from build123d import *

# Parameters (mm, degrees)
SKETCH2_R           = 5
BOSS_EXTRUDE1_DEPTH = 10


with BuildPart() as part:
    # Sketch2 → Boss-Extrude1 (new body)
    with BuildSketch(Plane(origin=(0, 0, 0), x_dir=(1, 0, 0), z_dir=(0, 1, 0))):
        with BuildLine():
            ThreePointArc((-27.5, -47.631397208), (-14.235047481, -53.125920446), (0, -55))
            add(Edge.make_bspline(
                [(0, -55), (15.821995191, -55.521684642), (37.158196695, -40.15721482), (40.409843735, -11.080588617), (32.003444862, 9.061174356), (19.786389501, 17.600648721), (12.5, 21.650635095)],
                knots=[0, 0, 0, 0, 0.421298926, 0.607822378, 0.766892621, 1, 1, 1, 1], degree=3))
            ThreePointArc((12.5, 21.650635095), (6.470476128, 24.148145657), (0, 25))
            add(Edge.make_bspline(
                [(0, 25), (-8.335191597, 25.135803666), (-23.185209081, 23.848929612), (-40.536245546, 10.608850636), (-52.258549707, -16.198069832), (-41.463092095, -40.172191766), (-27.5, -47.631397208)],
                knots=[0, 0, 0, 0, 0.233107379, 0.392177622, 0.578701074, 1, 1, 1, 1], degree=3))
        make_face()
        Circle(SKETCH2_R, mode=Mode.SUBTRACT)
    extrude(amount=BOSS_EXTRUDE1_DEPTH)


solid = part.part
Check sheet for the modelled part. Datum: model origin and axes. Units: mm. Round coordinates to 2 decimals unless told otherwise and drop trailing zeros. Return JSON: item names as keys, results as strings.
Q1. Draft check along Z on faces 1 (the cylindrical face through (-1.08, 4.93, 4.88)), 2 (the flat face through (-7, 0, 15)), 3 (the cylindrical face through (7, 5, -24)), 4 (the cylindrical face through (-14.43, 4.93, 53.073)). Enter one of: released by +Z, released by -Z, zero draft, split by the parting line, or undercut.
Returned:
{"face 1": "undercut", "face 2": "zero draft", "face 3": "released by -Z", "face 4": "released by +Z"}
Q2. Depth check by flat-ended pin: P1, Ø4, axis at y = 2.5, z = 8.5, coming from the +X side; P2, Ø2, axis at y = 6, z = 33, coming from the +X side; P3, Ø1.5, axis at y = 5, z = 16.5, coming from the -X side. Enter the tip coordinate at first touch or a pass-through.
Returned:
{"P1": "stops at x = 38.66", "P2": "stops at x = 35.76", "P3": "stops at x = -47.09"}
Q3. Scan lines: L1, parallel to X at y = 6.25, z = 0; L2, parallel to X at y = 3, z = 2; L3, parallel to X at y = 3, z = 40. Record each from-to range of solid material in increasing order. Write a range as from..to.
Returned:
{"L1": "x = -44.63..-5, 5..35.36", "L2": "x = -45.34..-4.58, 4.58..36.26", "L3": "x = -37.15..30.87"}
